```python
from build123d import *

# Parameters (mm, degrees)
SKETCH1_R           = 45
SKETCH1_R_2         = 9.55
SKETCH1_R_3         = 1.55
BOSS_EXTRUDE1_DEPTH = 5
SKETCH3_R           = 45
SKETCH3_R_2         = 5.25
SKETCH3_R_3         = 1.55
SKETCH3_R_4         = 1.347664629
SKETCH3_R_5         = 1.649528324
BOSS_EXTRUDE2_DEPTH = 5
SKETCH4_R           = 16
SKETCH4_R_2         = 10.1
BOSS_EXTRUDE3_DEPTH = 7
SKETCH5_R           = 1.525
CUT_EXTRUDE1_DEPTH  = 46
SKETCH8_R           = 3.275737446
CUT_EXTRUDE4_DEPTH  = 7


with BuildPart() as part:
    # Sketch1 → Boss-Extrude1 (new body)
    with BuildSketch(Plane(origin=(0, 0, 0), x_dir=(1, 0, 0), z_dir=(0, 1, 0))):
        Circle(SKETCH1_R)
        Circle(SKETCH1_R_2, mode=Mode.SUBTRACT)
        with Locations((23.534905201, -33.114037619)):
            Circle(SKETCH1_R_3, mode=Mode.SUBTRACT)
        with Locations((-16.9101452, -36.938844589)):
            Circle(SKETCH1_R_3, mode=Mode.SUBTRACT)
        with Locations((-40.4450504, -3.82480697)):
            Circle(SKETCH1_R_3, mode=Mode.SUBTRACT)
        with Locations((-23.534905201, 33.114037619)):
            Circle(SKETCH1_R_3, mode=Mode.SUBTRACT)
        with Locations((16.9101452, 36.938844589)):
            Circle(SKETCH1_R_3, mode=Mode.SUBTRACT)
        with Locations((40.4450504, 3.82480697)):
            Circle(SKETCH1_R_3, mode=Mode.SUBTRACT)
    extrude(amount=BOSS_EXTRUDE1_DEPTH)

    # Sketch3 → Boss-Extrude2 (add)
    with BuildSketch(Plane(origin=(0, 5, 0), x_dir=(1, 0, 0), z_dir=(0, 1, 0))):
        Circle(SKETCH3_R)
        Circle(SKETCH3_R_2, mode=Mode.SUBTRACT)
        with Locations((16.9101452, 36.938844589)):
            Circle(SKETCH3_R_3, mode=Mode.SUBTRACT)
        with Locations((40.4450504, 3.82480697)):
            Circle(SKETCH3_R_4, mode=Mode.SUBTRACT)
        with Locations((23.534905201, -33.114037619)):
            Circle(SKETCH3_R_3, mode=Mode.SUBTRACT)
        with Locations((-16.9101452, -36.938844589)):
            Circle(SKETCH3_R_5, mode=Mode.SUBTRACT)
        with Locations((-40.4450504, -3.82480697)):
            Circle(SKETCH3_R_3, mode=Mode.SUBTRACT)
        with Locations((-23.534905201, 33.114037619)):
            Circle(SKETCH3_R_3, mode=Mode.SUBTRACT)
    extrude(amount=BOSS_EXTRUDE2_DEPTH)

    # Sketch4 → Boss-Extrude3 (add)
    with BuildSketch(Plane(origin=(0, 10, 0), x_dir=(1, 0, 0), z_dir=(0, 1, 0))):
        Circle(SKETCH4_R)
        Circle(SKETCH4_R_2, mode=Mode.SUBTRACT)
    extrude(amount=BOSS_EXTRUDE3_DEPTH)

    # Sketch5 → Cut-Extrude1 (cut)
    with BuildSketch(Plane(origin=(0, 17, 0), x_dir=(1, 0, 0), z_dir=(0, 1, 0))):
        with Locations((12.786648762, 0)):
            Circle(SKETCH5_R)
        with Locations((-0.213351238, -13)):
            Circle(SKETCH5_R)
        with Locations((-13.213351238, 0)):
            Circle(SKETCH5_R)
        with Locations((-0.213351238, 13)):
            Circle(SKETCH5_R)
    extrude(amount=-CUT_EXTRUDE1_DEPTH, mode=Mode.SUBTRACT)

    # Sketch8 → Cut-Extrude4 (cut)
    with BuildSketch(Plane.XZ):
        with Locations((-0.213351238, -13)):
            Circle(SKETCH8_R)
        with Locations((-13, 0.213351238)):
            Circle(SKETCH8_R)
        with Locations((0.213351238, 13)):
            Circle(SKETCH8_R)
        with Locations((13, -0.213351238)):
            Circle(SKETCH8_R)
    extrude(amount=-CUT_EXTRUDE4_DEPTH, mode=Mode.SUBTRACT)


solid = part.part
```
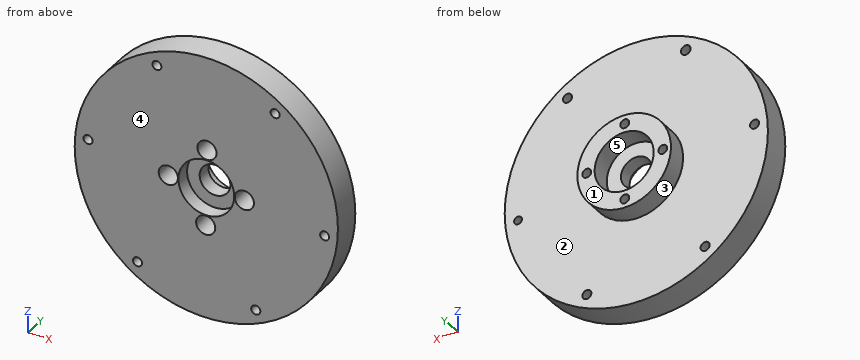
Check sheet for the modelled part. Datum: model origin and axes. Units: mm. Face numbers are marked on the shaded views. A direction names the side the tool comes from. Round coordinates to 2 decimals unless told otherwise and drop trailing zeros. Order: outer loops, then holes, each group sorted by start corner. A loop starts at its lowest first (then second) coordinate and runs counter-clockwise, first axis right, second up.
1) Scan lines: line 1 (Z direction, x = 0, y = 3.55); line 2 (X direction, y = 12.25, z = 0); line 3 (Z direction, x = 0, y = 14). Record each from-to range of solid material in increasing order.
2) Section check C-C (z = 13). Record the boundary of the cut face in (x, y).
3) Section check D-D (z = -7). Record the boundary of the cut face in (x, y), and give its area (3 significant figures).
4) Go/stop test with flat-tipped pins: pin 1 Ø3.5 at (x, z) = (-13.5, -1) entering from -Y; pin 2 Ø10 at (x, y) = (23.5, 6) entering from -Z; pin 3 Ø6 at (x, y) = (9, 5.5) entering from +Z. Record where each tip stops, or that it passes through.
5) Section check B-B (x = 13). Record the boundary of the cut face in (y, z), and give its area (3 significant figures).
6) Tool access check on the marked faces 1 and 2. Record the directions out of +Z, -Z, +X, -X, +Y, -Y that give a thin tool (end or side, any length) a straight path to the whole face; none if there is none.
7) Section check A-A (y = 8.25). Give the number of separate pieces and of enclosed holes in the cut face, and give its area (3 significant figures).
8) Mould release check, pull along Z, two halves, no side actions. Record for the marked faces 3, 4 and 5: +Z half, -Z half, draft (parallel to the pull), parting line (faces both ways), or undercut.
Result:
1. line 1: z = -45 to -16.27, -9.73 to -9.55, 9.55 to 9.73, 16.27 to 45
1. line 2: x = -16 to -14.74, -11.69 to -10.1, 10.1 to 11.26, 14.31 to 16
1. line 3: z = -16 to -14.51, -11.49 to -10.1, 10.1 to 11.49, 14.51 to 16
2. outline: (-43.08, 0) - (-3.06, 0) - (-3.06, 7) - (-1.74, 7) - (-1.74, 17) - (-9.33, 17) - (-9.33, 10) - (-43.08, 10) - close; (1.31, 7) - (3.49, 7) - (3.49, 0) - (43.08, 0) - (43.08, 10) - (9.33, 10) - (9.33, 17) - (1.31, 17) - close
3. outline: (-44.45, 0) - (-6.5, 0) - (-6.5, 5) - (6.5, 5) - (6.5, 0) - (44.45, 0) - (44.45, 10) - (14.39, 10) - (14.39, 17) - (7.28, 17) - (7.28, 10) - (-7.28, 10) - (-7.28, 17) - (-14.39, 17) - (-14.39, 10) - (-44.45, 10) - close
3. area: 924 mm2
4. pin 1: stops at y = 7
4. pin 2: stops at z = -41.02
4. pin 3: stops at z = 44.6
5. outline: (0, -43.08) - (10, -43.08) - (10, -9.33) - (17, -9.33) - (17, -1.51) - (7, -1.51) - (7, -3.49) - (0, -3.49) - close; (0, 3.06) - (7, 3.06) - (7, 1.51) - (17, 1.51) - (17, 9.33) - (10, 9.33) - (10, 43.08) - (0, 43.08) - close
5. area: 916 mm2
6. face 1: +Z, -Z, +X, -X, +Y
6. face 2: +Y
7. separate pieces: 1
7. enclosed holes: 11
7. area: 6,200 mm2
8. face 3: parting line
8. face 4: draft
8. face 5: undercut
